```python
from build123d import *

# Parameters (mm, degrees)
ESQUISSE1_R               = 1.5
T_LE_DE_BASE_PLI_E1_DEPTH = 3


# Sheet-metal steps are written as plain solids
with BuildPart() as part:
    # Esquisse1 → Tôle de base pliée1 (new body)
    with BuildSketch(Plane.XY):
        with BuildLine():
            Line((1154.170302219, 1982.451705153), (1153.201251986, 1974.007124545))
            Line((1153.201251986, 1974.007124545), (1156.579084229, 1973.619504452))
            ThreePointArc((1156.579084229, 1973.619504452), (1155.731717841, 1965.1750361), (1155.715622171, 1956.688174697))
            ThreePointArc((1155.715622171, 1956.688174697), (1162.175892986, 1949.303940909), (1170.827393014, 1953.931419154))
            ThreePointArc((1170.827393014, 1953.931419154), (1175.052398427, 1959.453694764), (1181.379439759, 1962.337225003))
            ThreePointArc((1181.379439759, 1962.337225003), (1192.728026875, 1963.512709412), (1204.119748438, 1962.879564131))
            Line((1204.119748438, 1962.879564131), (1204.957691875, 1970.181642657))
            Line((1204.957691875, 1970.181642657), (1207.441392054, 1969.896627882))
            Line((1207.441392054, 1969.896627882), (1208.171029877, 1976.25490034))
            Line((1208.171029877, 1976.25490034), (1204.991893648, 1976.619719251))
            Line((1204.991893648, 1976.619719251), (1205.276908423, 1979.10341943))
            Line((1205.276908423, 1979.10341943), (1203.533232527, 1979.303513385))
            Line((1203.533232527, 1979.303513385), (1203.248217753, 1976.819813206))
            Line((1203.248217753, 1976.819813206), (1201.757997646, 1976.990822071))
            Line((1201.757997646, 1976.990822071), (1202.04301242, 1979.47452225))
            Line((1202.04301242, 1979.47452225), (1196.578872027, 1980.101554754))
            Line((1196.578872027, 1980.101554754), (1196.293857252, 1977.617854575))
            Line((1196.293857252, 1977.617854575), (1188.445364687, 1978.518501263))
            Line((1188.445364687, 1978.518501263), (1188.046344003, 1975.041321013))
            Line((1188.046344003, 1975.041321013), (1172.945446915, 1976.774210843))
            Line((1172.945446915, 1976.774210843), (1173.3444676, 1980.251391093))
            Line((1173.3444676, 1980.251391093), (1167.383587171, 1980.935426552))
            Line((1167.383587171, 1980.935426552), (1167.668601945, 1983.419126731))
            Line((1167.668601945, 1983.419126731), (1158.727281302, 1984.445179919))
            Line((1158.727281302, 1984.445179919), (1158.442266527, 1981.961479741))
            Line((1158.442266527, 1981.961479741), (1154.170302219, 1982.451705153))
        make_face()
        with Locations((1163.512272203, 1957.725451963)):
            Circle(ESQUISSE1_R, mode=Mode.SUBTRACT)
    extrude(amount=-T_LE_DE_BASE_PLI_E1_DEPTH)


solid = part.part
```
Geometry: final body of the model. Coordinates: model frame, mm. A direction names the side the tool comes from. Give positions to 0.01 mm unless a question says otherwise; leave off trailing zeros. Order: outer loops, then holes, each group sorted by start corner. A loop starts at its lowest first (then second) coordinate and runs counter-clockwise, first axis right, second up. Notation, with made-up numbers: (4.25, 8.25) -> (26.25, 8.25) arc R17 cw to (26.25, 17.25) -> close; hole circle Ø5 at (62, 71.25). An arc over 180 degrees is marked (long way). Write each question's results on one line, items separated by ' | '. Start each with the question number.
1) Section A-A (z = -1.6). Return loops of the section in (x, y), then the cut area to 3 significant figures.
2) Section C-C (y = 1953). Return loops of the section in (x, z), then the cut area to 3 significant figures.
3) Section B-B (x = 1166). Return loops of the section in (y, z), then the cut area to 3 significant figures.
4) Line query: line 1 (X direction, y = 1959, z = -0.95); line 2 (X direction, y = 1975, z = -1.95); line 3 (X direction, y = 1958, z = -2.3). Output: solid intervals per line, ascending. Write a range as from..to.
5) Set-up query: faces 5 (the flat face through (1174, 1967, -3)), 6 (the flat face through (1201.9, 1978.22, -1.48)), 7 (the flat face through (1203.393, 1978.079, -1.479)). Return all of +Z, -Z, +X, -X, +Y, -Y with unobstructed straight access to the full face (end or side cutting, diameter ignored); none if empty.
6) Draft query along Y for faces 1 (the flat face through (1206.18, 1970.04, -1.48)), 2 (the flat face through (1205.13, 1977.84, -1.48)), 3 (the flat face through (1173.142, 1978.488, -1.479)), 4 (the flat face through (1199.349, 1979.784, -1.479)). Return one class per face: pulls with the +Y half, pulls with the -Y half, needs draft (parallel to the pull), parting line crosses it, or undercut.
7) First-contact query: pin 1 (1 mm diameter, centred on x = 1184.5, z = -1.5, fed in from +Y). Flat tip, straight axial feed; report the tip coordinate or a pass-through.
Calculated:
1) outline: (1153.2, 1974.01) -> (1156.58, 1973.62) arc R86.53 ccw to (1155.72, 1956.69) arc R7.88 ccw to (1170.83, 1953.93) arc R14.33 cw to (1181.38, 1962.34) arc R71.95 cw to (1204.12, 1962.88) -> (1204.96, 1970.18) -> (1207.44, 1969.9) -> (1208.17, 1976.25) -> (1204.99, 1976.62) -> (1205.28, 1979.1) -> (1203.53, 1979.3) -> (1203.25, 1976.82) -> (1201.76, 1976.99) -> (1202.04, 1979.47) -> (1196.58, 1980.1) -> (1196.29, 1977.62) -> (1188.45, 1978.52) -> (1188.05, 1975.04) -> (1172.95, 1976.77) -> (1173.34, 1980.25) -> (1167.38, 1980.94) -> (1167.67, 1983.42) -> (1158.73, 1984.45) -> (1158.44, 1981.96) -> (1154.17, 1982.45) -> close; hole circle Ø3 at (1163.51, 1957.73) | area: 1,040 mm2
2) outline: (1156.83, -3) -> (1170.35, -3) -> (1170.35, 0) -> (1156.83, 0) -> close | area: 40.5 mm2
3) outline: (1949.55, -3) -> (1983.61, -3) -> (1983.61, 0) -> (1949.55, 0) -> close | area: 102 mm2
4) line 1: 1155.64..1162.72, 1164.3..1174.51 | line 2: 1153.32..1208.03 | line 3: 1155.66..1162.04, 1164.99..1173.48
5) face 5: -Z, +X, -X, +Y, -Y | face 6: +Z, -Z | face 7: +Z, -Z, +Y
6) face 1: pulls with the -Y half | face 2: undercut | face 3: undercut | face 4: pulls with the +Y half
7) pin 1: y = 1975.51
